from build123d import *

# Parameters (mm, degrees)
CROQUIS1_W                         = 400
CROQUIS1_H                         = 38.1
SALIENTE_EXTRUIR1_DEPTH            = 9.525
TALADRO_DE_MARGEN_PARA_1_41_REACH  = 402.567
TALADRO_DE_MARGEN_PARA_1_41_BORE_R = 3.3782
TALADRO_ROSCADO_7_16_141_D         = 9.3472
TALADRO_ROSCADO_7_16_141_DEPTH     = 20
TALADRO_ROSCADO_7_16_141_TIP       = 2.808182189


with BuildPart() as part:
    # Croquis1 → Saliente-Extruir1 (new, symmetric)
    with BuildSketch(Plane.XY):
        Rectangle(CROQUIS1_W, CROQUIS1_H)
        with BuildLine():
            Line((-130, 6.35), (170, 6.35))
            ThreePointArc((170, 6.35), (176.35, 0), (170, -6.35))
            Line((170, -6.35), (-130, -6.35))
            ThreePointArc((-130, -6.35), (-136.35, 0), (-130, 6.35))
        make_face(mode=Mode.SUBTRACT)
    extrude(amount=SALIENTE_EXTRUIR1_DEPTH, both=True)

    # Taladro de margen para 1/41 bore → Taladro de margen para 1/41 (cut, up to next)
    with BuildSketch(Plane(origin=(200, 0, 0), x_dir=(0, 0, -1), z_dir=(1, 0, 0)), mode=Mode.PRIVATE) as taladro_de_margen_para_1_41_sk1:
        Circle(TALADRO_DE_MARGEN_PARA_1_41_BORE_R)
    taladro_de_margen_para_1_41_tool1 = extrude(taladro_de_margen_para_1_41_sk1.sketch, amount=-TALADRO_DE_MARGEN_PARA_1_41_REACH, mode=Mode.PRIVATE) & part.part
    add(taladro_de_margen_para_1_41_tool1.solids().sort_by_distance((200, 0, 0))[0], mode=Mode.SUBTRACT)

    # Taladro roscado 7/16-141
    with Locations(Plane.ZY.offset(200)):
        with Locations((0, 9), (0, -9)):
            Hole(TALADRO_ROSCADO_7_16_141_D / 2, depth=TALADRO_ROSCADO_7_16_141_DEPTH)
            with Locations((0, 0, -(TALADRO_ROSCADO_7_16_141_DEPTH + TALADRO_ROSCADO_7_16_141_TIP / 2))):  # 118° drill point
                Cone(0, TALADRO_ROSCADO_7_16_141_D / 2, TALADRO_ROSCADO_7_16_141_TIP, mode=Mode.SUBTRACT)


solid = part.part
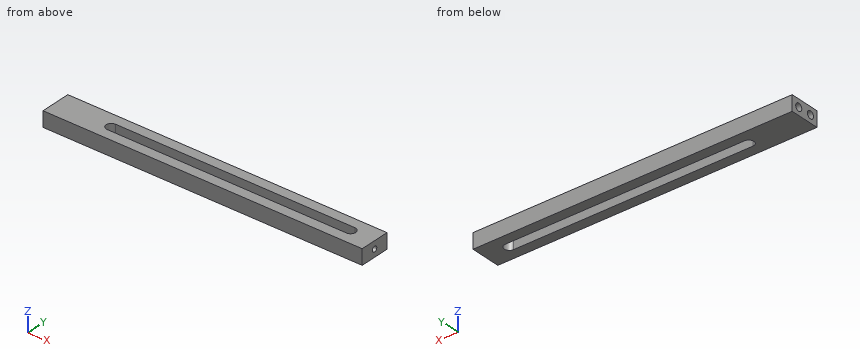
Work out the finished part from the listing and answer in its coordinate system (mm). Give positions to 0.01 mm unless a question says otherwise; leave off trailing zeros. Order: outer loops, then holes, each group sorted by start corner. A loop starts at its lowest first (then second) coordinate and runs counter-clockwise, first axis right, second up. Notation, with made-up numbers: M 66,67.5 L 84,67.5 A27 ccw 84,88.5 Z; hole C 31.25,21 d11. An arc over 180 degrees is marked long. Return JSON: item names as keys, results as strings.
Q1. Find the intervals of material crossed by line 1 along Y through (x, z) = (-189, 0); line 2 along Z through (x, y) = (-186.5, 9) (3 decimals); line 3 along Y through (x, z) = (83.5, 8.75), in increasing order. Write a range as [from, to].
Answer below:
{"line 1": "y = [-19.05, -13.67], [-4.33, 4.33], [13.67, 19.05]", "line 2": "z = [-9.525, -4.674], [4.674, 9.525]", "line 3": "y = [-19.05, -6.35], [6.35, 19.05]"}
Q2. Find section A-A, the plane x = -112. Write down the section's boundary in (y, z) (3 decimals).
Answer below:
{"outline": "M -19.05,-9.525 L -6.35,-9.525 L -6.35,9.525 L -19.05,9.525 Z; M 6.35,-9.525 L 19.05,-9.525 L 19.05,9.525 L 6.35,9.525 Z"}
Q3. Find section B-B, the plane y = 0. Write down the section's boundary in (x, z) (3 decimals).
Answer below:
{"outline": "M -200,-9.525 L -136.35,-9.525 L -136.35,9.525 L -200,9.525 Z; M 176.35,-9.525 L 200,-9.525 L 200,-3.378 L 176.35,-3.378 Z; M 176.35,3.378 L 200,3.378 L 200,9.525 L 176.35,9.525 Z"}
